Source: CAD feature listing. Evaluate the final solid. Frame: model axes, mm. A direction names the side the tool comes from. Coordinates: 2 decimals unless noted, no trailing zeros. Order: outer loops, then holes, each group sorted by start corner. A loop starts at its lowest first (then second) coordinate and runs counter-clockwise, first axis right, second up. Notation, with made-up numbers: (61, 5) -> (109, 5) arc R18 ccw to (109, 17) -> close; hole circle Ø1 at (26, 85). An arc over 180 degrees is marked (long way). Put each result on its own line as item: value.
from build123d import *

# Parameters (mm, degrees)
BOSS_EXTRUDE2_DEPTH = 300


with BuildPart() as part:
    # Sketch1 → Boss-Extrude2 (new body)
    with BuildSketch(Plane(origin=(0, 0, 0), x_dir=(1, 0, 0), z_dir=(0, 1, 0))):
        with BuildLine():
            Line((7, 57), (7, -57))
            Line((7, -57), (-63, -57))
            Line((-63, -57), (-63, -50))
            Line((-63, -50), (0, -50))
            Line((0, -50), (0, 50))
            Line((0, 50), (-63, 50))
            ThreePointArc((-63, 50), (-78.811388301, 47.434164903), (-93, 40))
            Line((-93, 40), (-105, 40))
            ThreePointArc((-105, 40), (-85.655021518, 52.588876693), (-63, 57))
            Line((-63, 57), (7, 57))
        make_face()
    extrude(amount=BOSS_EXTRUDE2_DEPTH)


solid = part.part
1. Cut plane B-B on y = 143.5. Output: boundary loops of the cut face in (x, z), plus the area to 3 significant figures.
Numbers:
outline: (-105, -40) arc R60.38 ccw to (-63, -57) -> (7, -57) -> (7, 57) -> (-63, 57) -> (-63, 50) -> (0, 50) -> (0, -50) -> (-63, -50) arc R50 cw to (-93, -40) -> close
area: 1,970 mm2
2. Cut plane A-A on x = -55.5. Output: boundary loops of the cut face in (y, z), plus the area to 3 significant figures.
Numbers:
outline: (0, -57) -> (300, -57) -> (300, -50) -> (0, -50) -> close; (0, 50) -> (300, 50) -> (300, 57) -> (0, 57) -> close
area: 4,200 mm2
3. Pull-direction query (Z, two-part tool) for faces 1 (the flat face through (-63, 148, 54)), 2 (the flat face through (-31, 148, -50)), 3 (the cylindrical face through (-78.598, 147.9, -47.505)), 4 (the flat face through (-32, 148, 50)); classes: pulls with the +Z half, pulls with the -Z half, needs draft (parallel to the pull), parting line crosses it, or undercut.
Numbers:
face 1: needs draft
face 2: undercut
face 3: pulls with the +Z half
face 4: undercut
4. Ray query, line 1 along Z through (x, y) = (-15.5, 180.5); line 2 along X through (y, z) = (229, 38); line 3 along X through (y, z) = (240, 50.5). Return the intervals inside material, ascending.
Numbers:
line 1: z = -57 to -50, 50 to 57
line 2: x = 0 to 7
line 3: x = -63 to 7
5. Set-up query: faces 5 (the flat face through (-99, 148, -40)), 6 (the flat face through (1, 0, -9)). Return all of +Z, -Z, +X, -X, +Y, -Y with unobstructed straight access to the full face (end or side cutting, diameter ignored); none if empty.
Numbers:
face 5: +Z, -X, +Y, -Y
face 6: +Z, -Z, +X, -X, -Y
6. First-contact query: pin 1 (3.5 mm diameter, centred on y = 82.5, z = 52, fed in from -X); pin 2 (12 mm diameter, centred on x = -78.5, y = 91.5, fed in from -Z); pin 3 (5 mm diameter, centred on y = 139, z = 20, fed in from -X). Flat tips, straight axial feed; report the tip coordinate or a pass-through.
Numbers:
pin 1: stops at x = -63
pin 2: stops at z = -56.25
pin 3: stops at x = 0
7. Cut plane C-C on z = -13. Output: boundary loops of the cut face in (x, y).
Numbers:
outline: (0, 0) -> (7, 0) -> (7, 300) -> (0, 300) -> close
8. Cut plane D-D on x = -75. Output: boundary loops of the cut face in (y, z), plus the area to 3 significant figures.
Numbers:
outline: (0, -55.8) -> (300, -55.8) -> (300, -48.54) -> (0, -48.54) -> close
area: 2,180 mm2
